The figure shows three views and two pictorial views of one solid part (mm, origin at its lowest corner). Answer the questions. A direction names the side the tool comes from. Coordinates: 2 decimals unless noted, no trailing zeros. Loops run counter-clockwise (first coordinate to the right, second up) from the corner with the lowest first, then second, coordinate; pieces in that order, holes last. Notation, with made-up numbers: M -7.75,28.25 L 43.25,28.25 A23 ccw 43.25,61.25 Z; hole C 85.5,51.5 d4. An arc over 180 degrees is marked long. Answer as a JSON object with one key per item and string values. Group by question number.
1. A cutting plane is placed at C-C on x = 36.25. Give the vertices of the cut face in (y, z), and give its area (3 significant figures).
2. A cutting plane is placed at A-A on y = 7.5. Give the vertices of the cut face in (x, z).
3. A cutting plane is placed at D-D on y = 10.5. Give the vertices of the cut face in (x, z).
4. Determine the mould class of the marked faces 3, 4 and 5 for opening direction X: released by +X, released by -X, zero draft, split by the parting line, or undercut.
5. Given pin 1 (4 mm diameter, centred on x = 18, z = 19, fed in from +Y); pin 2 (7.5 mm diameter, centred on x = 6.25, z = 7.35, fed in from +Y), each flat-ended and moving along its own axis, determine where each tip first touches the part or whether it passes through.
6. A cutting plane is placed at B-B on z = 31.65. Give the vertices of the cut face in (x, y).
7. For the marked faces 1 and 2, determine the directions among +Z, -Z, +X, -X, +Y, -Y from which every point of the face is accessible in a straight line to the end or side of a thin tool.
8. Straight lines are drawn through the part: L1, parallel to Z at x = 36.25, y = 5; L2, parallel to Z at x = 40, y = 7.5; L3, parallel to X at y = 5.25, z = 28.5. For each, find the intervals that lie inside material, in ascending order.
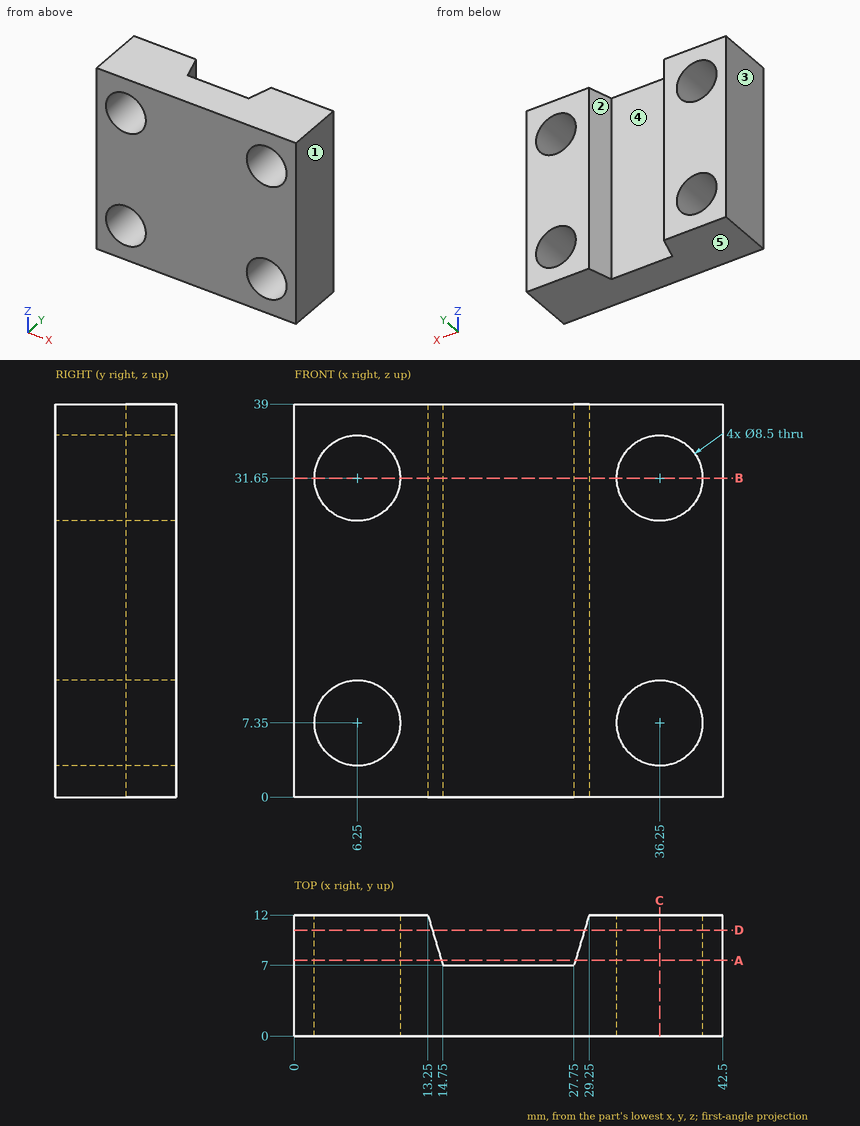
From the geometry:
{
 "1": {"outline": "M 0,0 L 12,0 L 12,3.1 L 0,3.1 Z; M 0,11.6 L 12,11.6 L 12,27.4 L 0,27.4 Z; M 0,35.9 L 12,35.9 L 12,39 L 0,39 Z", "area": "264 mm²"},
 "2": {"outline": "M 0,0 L 14.6,0 L 14.6,39 L 0,39 Z; M 27.9,0 L 42.5,0 L 42.5,39 L 27.9,39 Z; hole C 6.25,7.35 d8.5; hole C 6.25,31.65 d8.5; hole C 36.25,7.35 d8.5; hole C 36.25,31.65 d8.5"},
 "3": {"outline": "M 0,0 L 13.7,0 L 13.7,39 L 0,39 Z; M 28.8,0 L 42.5,0 L 42.5,39 L 28.8,39 Z; hole C 6.25,7.35 d8.5; hole C 6.25,31.65 d8.5; hole C 36.25,7.35 d8.5; hole C 36.25,31.65 d8.5"},
 "4": {"face 3": "released by -X", "face 4": "undercut", "face 5": "zero draft"},
 "5": {"pin 1": "stops at y = 7", "pin 2": "passes through"},
 "6": {"outline": "M 0,0 L 2,0 L 2,12 L 0,12 Z; M 10.5,0 L 32,0 L 32,12 L 29.25,12 L 27.75,7 L 14.75,7 L 13.25,12 L 10.5,12 Z; M 40.5,0 L 42.5,0 L 42.5,12 L 40.5,12 Z"},
 "7": {"face 1": "+Z, -Z, +X, +Y, -Y", "face 2": "+Z, -Z, +Y"},
 "8": {"L1": "z = 0 to 3.1, 11.6 to 27.4, 35.9 to 39", "L2": "z = 0 to 5.35, 9.35 to 29.65, 33.65 to 39", "L3": "x = 0 to 3.4, 9.1 to 33.4, 39.1 to 42.5"}
}
